```python
from build123d import *

# Parameters (mm, degrees)
SKETCH1_W           = 0.6
SKETCH1_H           = 0.6
BOSS_EXTRUDE1_DEPTH = 2.54


with BuildPart() as part:
    # Sketch1 → Boss-Extrude1 (new body)
    with BuildSketch(Plane(origin=(0, 0, 0), x_dir=(1, 0, 0), z_dir=(0, 1, 0))):
        Polygon((-0.5, 0), (-2.04, 0), (-2.54, 0.5), (-3.04, 0), (-4.58, 0), (-5.08, 0.5), (-5.08, 2.04), (-4.58, 2.54), (-3.04, 2.54), (-2.54, 2.04), (-2.04, 2.54), (-0.5, 2.54), (0, 2.04), (0.5, 2.54), (2.04, 2.54), (2.54, 2.04), (2.54, 0.5), (2.04, 0), (0.5, 0), (0, 0.5), align=None)
        with Locations((-3.81, 1.27)):
            Rectangle(SKETCH1_W, SKETCH1_H, mode=Mode.SUBTRACT)
        with Locations((-1.27, 1.27)):
            Rectangle(SKETCH1_W, SKETCH1_H, mode=Mode.SUBTRACT)
        with Locations((1.223573691, 1.27)):
            Rectangle(SKETCH1_W, SKETCH1_H, mode=Mode.SUBTRACT)
    extrude(amount=BOSS_EXTRUDE1_DEPTH)


solid = part.part
```
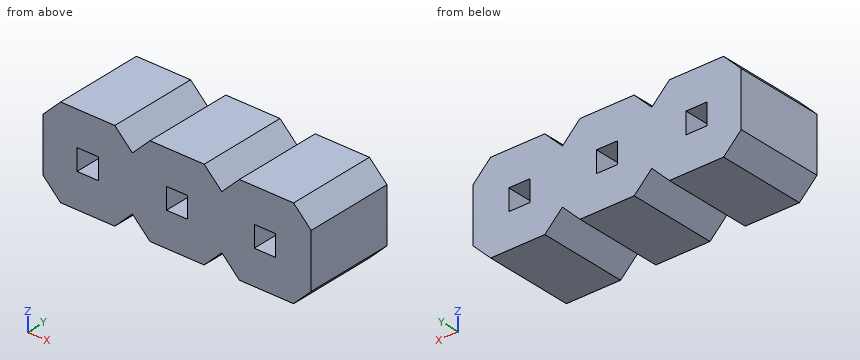
Read the model definition and answer for the solid it produces. Units are mm, in the model's axes. Give positions to 0.01 mm unless a question says otherwise; leave off trailing zeros. Loops run counter-clockwise (first coordinate to the right, second up) from the corner with the lowest first, then second, coordinate; pieces in that order, holes last.
Item 1: Find the intervals of material crossed by line 1 along X through (y, z) = (0.4, -1.25); line 2 along X through (y, z) = (1.3, -0.3); line 3 along Z through (x, y) = (-1.25, 1.9), in increasing order.
Item 2: The part is cut by section D-D (x = -0.25). Write down the section's boundary in (y, z), and give its area (3 significant figures).
Item 3: The part is cut by section C-C (y = 1.15). Give the number of separate pieces and of enclosed holes in the cut face, and give its area (3 significant figures).
Item 4: The part is cut by section B-B (z = -0.25). Write down the section's boundary in (x, y), and give its area (3 significant figures).
Item 5: The part is cut by section A-A (x = 1.25). Write down the section's boundary in (y, z).
Item 6: This flat-tipped pin is pushed along its axis until it touches: pin 1 Ø1 at (x, y) = (-2.5, 2) entering from +Z. Where does it stop, or does it pass through?
Taken from the geometry:
1. line 1: x = -5.08 to -4.11, -3.51 to -1.57, -0.97 to 0.92, 1.52 to 2.54
1. line 2: x = -4.88 to -2.74, -2.34 to -0.2, 0.2 to 2.34
1. line 3: z = -2.54 to -1.57, -0.97 to 0
2. outline: (0, -2.29) - (2.54, -2.29) - (2.54, -0.25) - (0, -0.25) - close
2. area: 5.18 mm2
3. separate pieces: 1
3. enclosed holes: 3
3. area: 16.8 mm2
4. outline: (-4.83, 0) - (-2.79, 0) - (-2.79, 2.54) - (-4.83, 2.54) - close; (-2.29, 0) - (-0.25, 0) - (-0.25, 2.54) - (-2.29, 2.54) - close; (0.25, 0) - (2.29, 0) - (2.29, 2.54) - (0.25, 2.54) - close
4. area: 15.5 mm2
5. outline: (0, -2.54) - (2.54, -2.54) - (2.54, -1.57) - (0, -1.57) - close; (0, -0.97) - (2.54, -0.97) - (2.54, 0) - (0, 0) - close
6. pin 1: stops at z = 0
